from build123d import *

# Parameters (mm, degrees)
F4_DEPTH = 5
F5_R     = 3


with BuildPart() as f2:
    # F1 (on Front) → F2 (revolve)
    with BuildSketch(Plane.XZ):
        with BuildLine():
            ThreePointArc((0, 1), (-2.44949, 2.267949), (-2.828427, 5))
            Line((-2.828427, 5), (-4, 5))
            Line((-4, 5), (-4, 0))
            Line((-4, 0), (0, 0))
            Line((0, 0), (0, 1))
        make_face()
    revolve(axis=Axis((0, 0, -0.010433), (0, 0, -1)))

    # F3 (on Top) → F4 (join)
    with BuildSketch(Plane.XY):
        with BuildLine():
            ThreePointArc((0, -4), (-2.828427, -2.828427), (-4, 0))
            Line((-4, 0), (-4, -4))
            Line((-4, -4), (0, -4))
        make_face()
        with BuildLine():
            Line((4, -4), (4, 0))
            ThreePointArc((4, 0), (2.828427, -2.828427), (0, -4))
            Line((0, -4), (4, -4))
        make_face()
        with BuildLine():
            Line((4, 4), (0, 4))
            ThreePointArc((0, 4), (2.828427, 2.828427), (4, 0))
            Line((4, 0), (4, 4))
        make_face()
        with BuildLine():
            Line((0, 4), (-4, 4))
            Line((-4, 4), (-4, 0))
            ThreePointArc((-4, 0), (-2.828427, 2.828427), (0, 4))
        make_face()
    extrude(amount=F4_DEPTH)

    # F5
    f5_edges = [f2.edges().sort_by_distance(p)[0] for p in [
        (4, -4, 2.5),
        (4, 4, 2.5),
        (-4, -4, 2.5),
        (-4, 4, 2.5),
    ]]
    fillet(f5_edges, radius=F5_R)


solid = f2.part
Geometry: final body of the model. Coordinates: model frame, mm. Coordinates: 2 decimals unless noted, no trailing zeros. Loops run counter-clockwise (first coordinate to the right, second up) from the corner with the lowest first, then second, coordinate; pieces in that order, holes last. Notation, with made-up numbers: (89.25, 9) - (100.25, 9) arc R20 cw to (100.25, 13) - close; hole circle Ø2 at (35.5, -10.5). An arc over 180 degrees is marked (long way). Put each result on its own line as item: value. Start each with the question number.
Q1. Pin query (flat end, axial travel): pin 1 Ø2 at (x, z) = (1.5, 2.5) entering from -Y. Return the tip coordinate at first contact, or that it passes through.
Q2. Line query: line 1 (X direction, y = 2, z = 4); line 2 (Y direction, x = -2.25, z = 4.5); line 3 (X direction, y = -0.75, z = 3.7). Output: solid intervals per line, ascending.
Q3. Cut plane A-A, the plane z = 0.45. Return loops of the section in (x, y).
Q4. Cut plane B-B, the plane y = -3.5. Return loops of the section in (x, z).
Filled sheet:
1. pin 1: y = -4
2. line 1: -3.83 to -2.24, 2.24 to 3.83
2. line 2: -3.73 to -1.92, 1.92 to 3.73
2. line 3: -4 to -2.89, 2.89 to 4
3. outline: (-4, -1) arc R3 ccw to (-1, -4) - (1, -4) arc R3 ccw to (4, -1) - (4, 1) arc R3 ccw to (1, 4) - (-1, 4) arc R3 ccw to (-4, 1) - close
4. outline: (-2.66, 0) - (2.66, 0) - (2.66, 5) - (-2.66, 5) - close
